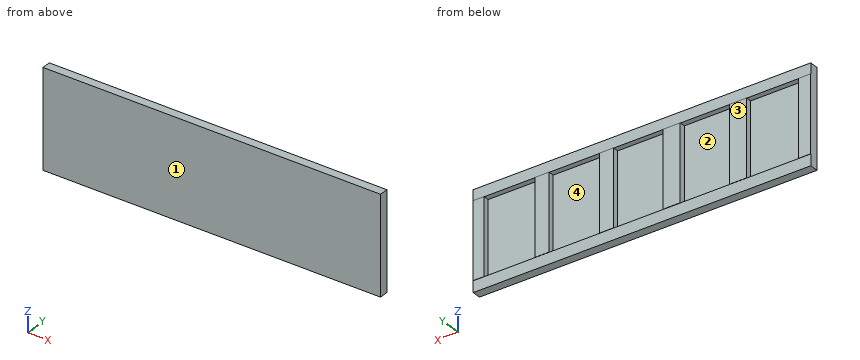
```python
from build123d import *

# Parameters (mm, degrees)
F0_W      = 787.3788177967
F0_H      = 229.1885906598
F1_DEPTH  = 7.62
F2_W      = 787.3788177967
F2_H      = 24.8994113645
F3_DEPTH  = 12.7
F4_W      = 787.3788177967
F4_H      = 26.2663476169
F5_DEPTH  = 12.7
F6_W      = 25.7195234299
F6_H      = 178.0228316784
F7_DEPTH  = 13.462
F8_W      = 27.5898575783
F8_H      = 178.0228316784
F9_DEPTH  = 13.462
F10_W     = 32.9714715481
F10_H     = 178.0228316784
F11_DEPTH = 13.462
F12_W     = 32.9747404903
F12_H     = 178.0228316784
F13_DEPTH = 13.462
F14_W     = 39.5713537
F14_H     = 178.0228316784
F15_DEPTH = 13.462
F16_W     = 39.5713876933
F16_H     = 178.0228316784
F17_DEPTH = 13.462


with BuildPart() as f1:
    # F0 (on Front) → F1 (new body)
    with BuildSketch(Plane.XZ):
        with Locations((43.1885272264, 1.5531365643)):
            Rectangle(F0_W, F0_H)
    extrude(amount=F1_DEPTH)

    # F2 (on face) → F3 (join)
    with BuildSketch(Plane(origin=(0, 0, 0), x_dir=(-1, 0, 0), z_dir=(0, 1, 0))):
        with Locations((-43.1885272264, 103.697726212)):
            Rectangle(F2_W, F2_H)
    extrude(amount=F3_DEPTH)

    # F4 (on face) → F5 (join)
    with BuildSketch(Plane(origin=(0, 0, 0), x_dir=(-1, 0, 0), z_dir=(0, 1, 0))):
        with Locations((-43.1885272264, -99.9079849571)):
            Rectangle(F4_W, F4_H)
    extrude(amount=F5_DEPTH)

    # F6 (on face) → F7 (join)
    with BuildSketch(Plane(origin=(0, 0, 0), x_dir=(-1, 0, 0), z_dir=(0, 1, 0))):
        with Locations((-424.0181744099, 2.2366046906)):
            Rectangle(F6_W, F6_H)
    extrude(amount=F7_DEPTH)

    # F8 (on face) → F9 (join)
    with BuildSketch(Plane(origin=(0, 0, 0), x_dir=(-1, 0, 0), z_dir=(0, 1, 0))):
        with Locations((336.7059528828, 2.2366046906)):
            Rectangle(F8_W, F8_H)
    extrude(amount=F9_DEPTH)

    # F10 (on face) → F11 (join)
    with BuildSketch(Plane(origin=(0, 0, 0), x_dir=(-1, 0, 0), z_dir=(0, 1, 0))):
        with Locations((-275.9774178267, 2.2366046906)):
            Rectangle(F10_W, F10_H)
    extrude(amount=F11_DEPTH)

    # F12 (on face) → F13 (join)
    with BuildSketch(Plane(origin=(0, 0, 0), x_dir=(-1, 0, 0), z_dir=(0, 1, 0))):
        with Locations((-125.517684035, 2.2366046906)):
            Rectangle(F12_W, F12_H)
    extrude(amount=F13_DEPTH)

    # F14 (on face) → F15 (join)
    with BuildSketch(Plane(origin=(0, 0, 0), x_dir=(-1, 0, 0), z_dir=(0, 1, 0))):
        with Locations((26.6765605193, 2.2366046906)):
            Rectangle(F14_W, F14_H)
    extrude(amount=F15_DEPTH)

    # F16 (on face) → F17 (join)
    with BuildSketch(Plane(origin=(0, 0, 0), x_dir=(-1, 0, 0), z_dir=(0, 1, 0))):
        with Locations((181.3858910464, 2.2366046906)):
            Rectangle(F16_W, F16_H)
    extrude(amount=F17_DEPTH)


solid = f1.part
```
The model under review builds one solid part; all positions refer to its coordinate system, in mm. Face numbers are marked on the shaded views. A direction names the side the tool comes from. Round coordinates to 2 decimals unless told otherwise and drop trailing zeros. Order: outer loops, then holes, each group sorted by start corner. A loop starts at its lowest first (then second) coordinate and runs counter-clockwise, first axis right, second up. Notation, with made-up numbers: (71.25, 67.25) -> (107.25, 67.25) arc R8 ccw to (107.25, 73.25) -> close; hole circle Ø7 at (-2, 13). An arc over 180 degrees is marked (long way). Use a Markdown table: item, result.
Q1. We need section B-B on x = 219. Write out the cut boundary in (y, z).
Values:
| item | result |
|---|---|
| outline | (-7.62, -113.04) -> (12.7, -113.04) -> (12.7, -86.77) -> (0, -86.77) -> (0, 91.25) -> (12.7, 91.25) -> (12.7, 116.15) -> (-7.62, 116.15) -> close |
Q2. For line 1 (X direction, y = 5.75, z = -39); line 2 (Z direction, x = 144.5, y = 8.75); line 3 (Y direction, x = -146.5, z = -86), list the stretches that pass through material, from the lowest coordinate up.
Values:
| item | result |
|---|---|
| line 1 | x = -350.5 to -322.91, -201.17 to -161.6, -46.46 to -6.89, 109.03 to 142.01, 259.49 to 292.46, 411.16 to 436.88 |
| line 2 | z = -113.04 to -86.77, 91.25 to 116.15 |
| line 3 | y = -7.62 to 0 |
Q3. Tool access review of the marked faces 1 and 2: name each direction out of +Z, -Z, +X, -X, +Y, -Y from which nothing blocks a thin tool from reaching the whole face with its end or side.
Values:
| item | result |
|---|---|
| face 1 | +Z, -Z, +X, -X, -Y |
| face 2 | +Y |
Q4. We need section A-A on z = 33.5. Write out the cut boundary in (x, y).
Values:
| item | result |
|---|---|
| outline | (-350.5, -7.62) -> (436.88, -7.62) -> (436.88, 13.46) -> (411.16, 13.46) -> (411.16, 0) -> (292.46, 0) -> (292.46, 13.46) -> (259.49, 13.46) -> (259.49, 0) -> (142.01, 0) -> (142.01, 13.46) -> (109.03, 13.46) -> (109.03, 0) -> (-6.89, 0) -> (-6.89, 13.46) -> (-46.46, 13.46) -> (-46.46, 0) -> (-161.6, 0) -> (-161.6, 13.46) -> (-201.17, 13.46) -> (-201.17, 0) -> (-322.91, 0) -> (-322.91, 13.46) -> (-350.5, 13.46) -> close |
Q5. We need section C-C on y = 4.5. Write out the cut boundary in (x, z), then the cut area to 3 significant figures.
Values:
| item | result |
|---|---|
| outline | (-350.5, -113.04) -> (436.88, -113.04) -> (436.88, 116.15) -> (-350.5, 116.15) -> close; hole (-322.91, -86.77) -> (-201.17, -86.77) -> (-201.17, 91.25) -> (-322.91, 91.25) -> close; hole (-161.6, -86.77) -> (-46.46, -86.77) -> (-46.46, 91.25) -> (-161.6, 91.25) -> close; hole (-6.89, -86.77) -> (109.03, -86.77) -> (109.03, 91.25) -> (-6.89, 91.25) -> close; hole (142.01, -86.77) -> (259.49, -86.77) -> (259.49, 91.25) -> (142.01, 91.25) -> close; hole (292.46, -86.77) -> (411.16, -86.77) -> (411.16, 91.25) -> (292.46, 91.25) -> close |
| area | 75,600 mm^2 |
Q6. Mouldability with a two-part tool opening along X and no side actions: class the marked faces 3 and 4 as +X half, -X half, draft (parallel to the pull), parting line (faces both ways), or undercut.
Values:
| item | result |
|---|---|
| face 3 | draft |
| face 4 | undercut |
